from build123d import *

# Parameters (mm, degrees)
BOSS_EXTRU_1_DEPTH      = 25
ENL_V_MAT_EXTRU_1_DEPTH = 26
ESQUISSE13_R            = 1.7
ENL_V_MAT_EXTRU_2_DEPTH = 29


with BuildPart() as part:
    # Esquisse1 → Boss.-Extru.1 (new body)
    with BuildSketch(Plane.XY.offset(25)):
        with BuildLine():
            Line((18.085571367, -30.291755058), (32.51257447, -26.185469451))
            ThreePointArc((32.51257447, -26.185469451), (36.161897649, -26.608505924), (38.443226857, -29.48809905))
            Line((38.443226857, -29.48809905), (44.28142645, -50))
            Line((44.28142645, -50), (-44.28142645, -50))
            Line((-44.28142645, -50), (-38.443226857, -29.48809905))
            ThreePointArc((-38.443226857, -29.48809905), (-36.161897649, -26.608505924), (-32.51257447, -26.185469451))
            Line((-32.51257447, -26.185469451), (-18.085571367, -30.291755058))
            ThreePointArc((-18.085571367, -30.291755058), (-9.130400918, -32.181477949), (0, -32.81544125))
            ThreePointArc((0, -32.81544125), (9.130400918, -32.181477949), (18.085571367, -30.291755058))
        make_face()
    extrude(amount=-BOSS_EXTRU_1_DEPTH)

    # Esquisse2 → Enlèv. mat.-Extru.1 (cut, through all)
    with BuildSketch(Plane(origin=(0, 0, 0), x_dir=(-1, 0, 0), z_dir=(0, 0, -1))):
        with BuildLine():
            Line((-10, -44), (10, -44))
            ThreePointArc((10, -44), (14, -40), (10, -36))
            Line((10, -36), (-10, -36))
            ThreePointArc((-10, -36), (-14, -40), (-10, -44))
        make_face()
    extrude(amount=-ENL_V_MAT_EXTRU_1_DEPTH, mode=Mode.SUBTRACT)

    # Esquisse13 → Enlèv. mat.-Extru.2 (cut, through all)
    with BuildSketch(Plane(origin=(0, 0, -3), x_dir=(-1, 0, 0), z_dir=(0, 0, -1))):
        with Locations((31.669980911, -35)):
            Circle(ESQUISSE13_R)
        with Locations((-31.669980911, -35)):
            Circle(ESQUISSE13_R)
    extrude(amount=-ENL_V_MAT_EXTRU_2_DEPTH, mode=Mode.SUBTRACT)


solid = part.part
Source: CAD feature listing. Evaluate the final solid. Frame: model axes, mm. A direction names the side the tool comes from. Round coordinates to 2 decimals unless told otherwise and drop trailing zeros. Loops run counter-clockwise (first coordinate to the right, second up) from the corner with the lowest first, then second, coordinate; pieces in that order, holes last.
Q1. Section D-D, the plane z = 18.75. Return loops of the section in (x, y), plus the area to 3 significant figures.
Q2. Access query for faces 1 (the face through (1, -50, 13)), 2 (the face through (-14, -40, 12)), 3 (the face through (-25.4, -28.21, 12.68)). Directions: +Z, -Z, +X, -X, +Y, -Y. A direction counts if a zero-diameter tool reaches every point of the face in a straight line with its end or side. Return the directions, or none.
Q3. Section A-A, the plane y = -28.5. Return loops of the section in (x, z), plus the area to 3 significant figures.
Q4. Mould query, pull axis Y, two halves, no side actions, for faces 4 (the face through (-32.45, -36.51, 12.32)), 5 (the face through (-36.208, -26.634, 12.675)), 6 (the face through (1, -35, 0)). Classes: pulls with the +Y half, pulls with the -Y half, needs draft (parallel to the pull), parting line crosses it, or undercut.
Q5. Ray query, line 1 (X direction, y = -33.5, z = 15); line 2 (Y direction, x = -9, z = 10); line 3 (Y direction, x = -11, z = 15.25). Return the intervals inside material, ascending.
Q6. Section B-B, the plane x = 31. Return loops of the section in (y, z).
Q7. First-contact query: P1, Ø10, axis at x = 0.5, z = 14, coming from the +Y side; P2, Ø5, axis at x = -5, z = 3.5, coming from the +Y side; P3, Ø6, axis at x = -0.5, z = 12, coming from the +Y side. Flat tips, straight axial feed; report the tip coordinate or a pass-through.
Q8. Section C-C, the plane y = -35. Return loops of the section in (x, z).
Solutions:
1. outline: (-44.28, -50) - (44.28, -50) - (38.44, -29.49) arc R4.8 ccw to (32.51, -26.19) - (18.09, -30.29) arc R66.07 cw to (-18.09, -30.29) - (-32.51, -26.19) arc R4.8 ccw to (-38.44, -29.49) - close; hole circle Ø3.4 at (-31.67, -35); hole (-10, -44) - (10, -44) arc R4 ccw to (10, -36) - (-10, -36) arc R4 ccw to start; hole circle Ø3.4 at (31.67, -35)
1. area: 1,450 mm2
2. face 1: +Z, -Z, +X, -X, -Y
2. face 2: +Z, -Z
2. face 3: +Z, -Z, +Y
3. outline: (-38.04, 0) - (-24.38, 0) - (-24.38, 25) - (-38.04, 25) - close; (24.38, 0) - (38.04, 0) - (38.04, 25) - (24.38, 25) - close
3. area: 683 mm2
4. face 4: undercut
4. face 5: pulls with the +Y half
4. face 6: needs draft
5. line 1: x = -39.59 to -32.47, -30.87 to 30.87, 32.47 to 39.59
5. line 2: y = -50 to -44, -36 to -32.2
5. line 3: y = -50 to -43.87, -36.13 to -31.89
6. outline: (-50, 0) - (-36.56, 0) - (-36.56, 25) - (-50, 25) - close; (-33.44, 0) - (-26.62, 0) - (-26.62, 25) - (-33.44, 25) - close
7. P1: stops at y = -32.59
7. P2: stops at y = -32.39
7. P3: stops at y = -32.72
8. outline: (-40.01, 0) - (-33.37, 0) - (-33.37, 25) - (-40.01, 25) - close; (-29.97, 0) - (29.97, 0) - (29.97, 25) - (-29.97, 25) - close; (33.37, 0) - (40.01, 0) - (40.01, 25) - (33.37, 25) - close
